Can you work these out from the model? Positions are in its coordinate system, mm. Face numbers are marked on the shaded views. A direction names the side the tool comes from. Round coordinates to 2 decimals unless told otherwise and drop trailing zeros. Loops run counter-clockwise (first coordinate to the right, second up) from the corner with the lowest first, then second, coordinate; pieces in that order, holes last. Notation, with made-up numbers: M -39,-39.75 L -22,-39.75 A9 cw -22,-32.75 Z; hole C 62,43 d4. An arc over 180 degrees is marked long. Use a Markdown table: item, result. Add a question column.
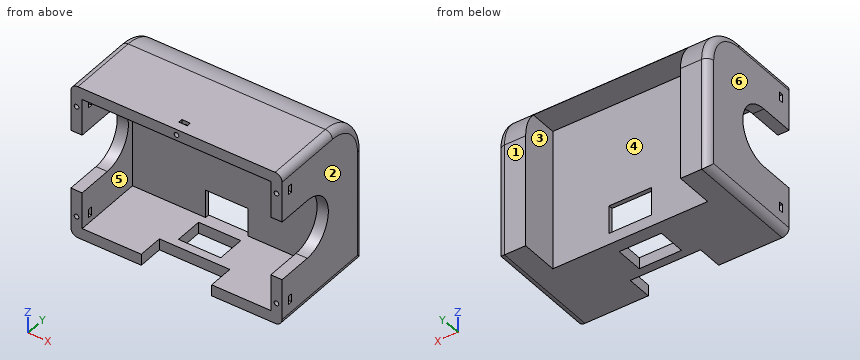
```python
from build123d import *

# Parameters (mm, degrees)
SKETCH_1_W          = 150
SKETCH_1_H          = 110
EXTRUDE_1_DEPTH     = 80
FILLET_3_R          = 30
FILLET_1_R          = 5
CUT_EXTRUDE_1_DEPTH = 151
SKETCH_3_W          = 50
SKETCH_3_H          = 18
CUT_EXTRUDE_2_DEPTH = 50
SKETCH_4_W          = 134
SKETCH_4_H          = 94
CUT_EXTRUDE_3_DEPTH = 50
SKETCH_5_W          = 110
SKETCH_5_H          = 100
CUT_EXTRUDE_4_DEPTH = 27
SKETCH_6_W          = 30
SKETCH_6_H          = 20
CUT_EXTRUDE_5_DEPTH = 23.3
SKETCH_7_W          = 30
SKETCH_7_H          = 20
CUT_EXTRUDE_6_DEPTH = 23.3
SKETCH_8_R          = 1.65
CUT_EXTRUDE_7_DEPTH = 10
SKETCH_11_W         = 6
SKETCH_11_H         = 3
CUT_EXTRUDE_8_DEPTH = 161
SKETCH_12_W         = 6
SKETCH_12_H         = 3
CUT_EXTRUDE_9_DEPTH = 161


with BuildPart() as part:
    # 草图1 → 凸台-拉伸1 (new body)
    with BuildSketch(Plane(origin=(0, 0, 0), x_dir=(1, 0, 0), z_dir=(0, 1, 0))):
        Rectangle(SKETCH_1_W, SKETCH_1_H)
    extrude(amount=EXTRUDE_1_DEPTH)

    # 圆角3
    fillet_3_edges = [part.edges().sort_by_distance(p)[0] for p in [
        (0, 80, 55),
    ]]
    fillet(fillet_3_edges, radius=FILLET_3_R)

    # 圆角1
    fillet_1_edges = [part.edges().sort_by_distance(p)[0] for p in [
        (-75, 80, -15),
        (75, 80, -15),
        (75, 25, 55),
        (75, 71.213203436, 46.213203436),
        (-75, 25, 55),
        (-75, 71.213203436, 46.213203436),
        (-75, 40, -55),
        (75, 40, -55),
    ]]
    fillet(fillet_1_edges, radius=FILLET_1_R)

    # 草图2 → 切除-拉伸1 (cut, through all)
    with BuildSketch(Plane(origin=(75, 0, 0), x_dir=(0, 0, -1), z_dir=(1, 0, 0))):
        with BuildLine():
            Line((-21, 25), (-21, 0))
            Line((-21, 0), (21, 0))
            Line((21, 0), (21, 25))
            ThreePointArc((21, 25), (0, 46), (-21, 25))
        make_face()
    extrude(amount=-CUT_EXTRUDE_1_DEPTH, mode=Mode.SUBTRACT)

    # 草图3 → 切除-拉伸2 (cut)
    with BuildSketch(Plane(origin=(0, 0, -55), x_dir=(-1, 0, 0), z_dir=(0, 0, -1))):
        with Locations((0, 9)):
            Rectangle(SKETCH_3_W, SKETCH_3_H)
    extrude(amount=-CUT_EXTRUDE_2_DEPTH, mode=Mode.SUBTRACT)

    # 草图4 → 切除-拉伸3 (cut)
    with BuildSketch(Plane.XZ):
        Rectangle(SKETCH_4_W, SKETCH_4_H)
    extrude(amount=-CUT_EXTRUDE_3_DEPTH, mode=Mode.SUBTRACT)

    # 草图5 → 切除-拉伸4 (cut)
    with BuildSketch(Plane(origin=(0, 80, 0), x_dir=(1, 0, 0), z_dir=(0, 1, 0))):
        with Locations((0, 5)):
            Rectangle(SKETCH_5_W, SKETCH_5_H)
    extrude(amount=-CUT_EXTRUDE_4_DEPTH, mode=Mode.SUBTRACT)

    # 草图6 → 切除-拉伸5 (cut)
    with BuildSketch(Plane(origin=(0, 0, -55), x_dir=(-1, 0, 0), z_dir=(0, 0, -1))):
        with Locations((0.741149686, 34)):
            Rectangle(SKETCH_6_W, SKETCH_6_H)
    extrude(amount=-CUT_EXTRUDE_5_DEPTH, mode=Mode.SUBTRACT)

    # 草图7 → 切除-拉伸6 (cut)
    with BuildSketch(Plane(origin=(0, 53, 0), x_dir=(1, 0, 0), z_dir=(0, 1, 0))):
        with Locations((0, 37)):
            Rectangle(SKETCH_7_W, SKETCH_7_H)
    extrude(amount=-CUT_EXTRUDE_6_DEPTH, mode=Mode.SUBTRACT)

    # 草图8 → 切除-拉伸7 (cut)
    with BuildSketch(Plane.XZ):
        with Locations((71, 40)):
            Circle(SKETCH_8_R)
        with Locations((71, -40)):
            Circle(SKETCH_8_R)
        with Locations((-71, -40)):
            Circle(SKETCH_8_R)
        with Locations((-71, 40)):
            Circle(SKETCH_8_R)
        with Locations((0, 51)):
            Circle(SKETCH_8_R)
    extrude(amount=-CUT_EXTRUDE_7_DEPTH, mode=Mode.SUBTRACT)

    # 草图11 → 切除-拉伸8 (cut)
    with BuildSketch(Plane.ZY.offset(75)):
        with Locations((-40, 8)):
            Rectangle(SKETCH_11_W, SKETCH_11_H)
        with Locations((40, 8)):
            Rectangle(SKETCH_11_W, SKETCH_11_H)
    extrude(amount=-CUT_EXTRUDE_8_DEPTH, mode=Mode.SUBTRACT)

    # 草图12 → 切除-拉伸9 (cut)
    with BuildSketch(Plane.XY.offset(55)):
        with Locations((0, 8)):
            Rectangle(SKETCH_12_W, SKETCH_12_H)
    extrude(amount=-CUT_EXTRUDE_9_DEPTH, mode=Mode.SUBTRACT)


solid = part.part
```
(1) Suppose I cut it at D-D on z = -40. Count the separate pieces of the cut face and the enclosed holes in it, and give its area (3 significant figures).
(2) On a 3-axis mill with a long thin cutter (end or side, diameter ignored), from which of +Z, -Z, +X, -X, +Y, -Y can I reach the whole of each face in a straight line? I mean the marked faces 4, 5 and 6. Say none if no direction works.
(3) Suppose I cut it at A-A on x = 0. List the corners of the cut face in (y, z) for me.
(4) Thinking about a two-plate mould opening in X: for the marked faces 1, 2 and 3, which applies, released by +X, released by -X, zero draft, split by the parting line, or undercut?
(5) Suppose I cut it at B-B on z = 0. List the corners of the cut face in (x, y) for me.
(6) I'm going to push flat-ended pins straight in: pin 1 (5 mm diameter, centred on x = 69.5, z = -39, fed in from -Y); pin 2 (1.5 mm diameter, centred on x = -37.5, z = -19.5, fed in from -Y); pin 3 (1.5 mm diameter, centred on x = -71, y = 8.5, fed in from -Z); pin 4 (3 mm diameter, centred on x = 46, z = 0, fed in from +Y). Where does each tip first touch, or does it pass through?
(7) If I drill on probe 1 along Z at (x, y) = (-20, 40); probe 2 along Z at (x, y) = (-71, 9.75); probe 3 along X at (y, z) = (28, 34.5), over which ranges is the centre line in solid material (lowest first)? Write a range as [from, to].
(8) Suppose I cut it at C-C on x = 30. List the corners of the cut face in (y, z) for me, and give its area (3 significant figures).
Results below:
| question | item | result |
|---|---|---|
| 1 | separate pieces | 6 |
| 1 | enclosed holes | 0 |
| 1 | area | 2,140 mm² |
| 2 | face 4 | -Z, +Y |
| 2 | face 5 | -Y |
| 2 | face 6 | +Z, -Z, -X, +Y, -Y |
| 3 | outline | M 0,47 L 6.5,47 L 6.5,49.35 L 0,49.35 Z; M 0,52.65 L 6.5,52.65 L 6.5,55 L 0,55 Z; M 9.5,47 L 50,47 L 50,-27 L 53,-27 L 53,45 L 72.36,45 A30 ccw 50,55 L 9.5,55 L 9.5,52.65 L 10,52.65 L 10,49.35 L 9.5,49.35 Z; M 18,-55 L 24,-55 L 24,-47 L 18,-47 Z; M 44,-55 L 53,-55 L 53,-47 L 44,-47 Z |
| 4 | face 1 | zero draft |
| 4 | face 2 | released by +X |
| 4 | face 3 | undercut |
| 5 | outline | M -75,46 L -67,46 L -67,50 L 67,50 L 67,46 L 75,46 L 75,75 A5 ccw 70,80 L 55,80 L 55,53 L -55,53 L -55,80 L -70,80 A5 ccw -75,75 Z |
| 6 | pin 1 | stops at y = 0 |
| 6 | pin 2 | stops at y = 50 |
| 6 | pin 3 | stops at z = -54.99 |
| 6 | pin 4 | stops at y = 53 |
| 7 | probe 1 | z = [-55, -47], [47, 55] |
| 7 | probe 2 | z = [-54.9, -41.65], [-38.35, -21], [21, 38.35], [41.65, 54.9] |
| 7 | probe 3 | x = [-75, -67], [67, 75] |
| 8 | outline | M 0,-55 L 53,-55 L 53,45 L 72.36,45 A30 ccw 50,55 L 0,55 L 0,47 L 50,47 L 50,-47 L 0,-47 Z |
| 8 | area | 1,250 mm² |
